Can you work these out from the model? Positions are in its coordinate system, mm. Face numbers are marked on the shaded views. A direction names the side the tool comes from. Give positions to 0.01 mm unless a question says otherwise; leave off trailing zeros. Order: outer loops, then holes, each group sorted by start corner. A loop starts at its lowest first (then second) coordinate and runs counter-clockwise, first axis right, second up. Notation, with made-up numbers: (87, -3.5) - (137, -3.5) arc R25 ccw to (137, 22.5) - close; hole circle Ø6 at (50.25, 7). An arc over 180 degrees is marked (long way). Answer as CSV lines item,"result".
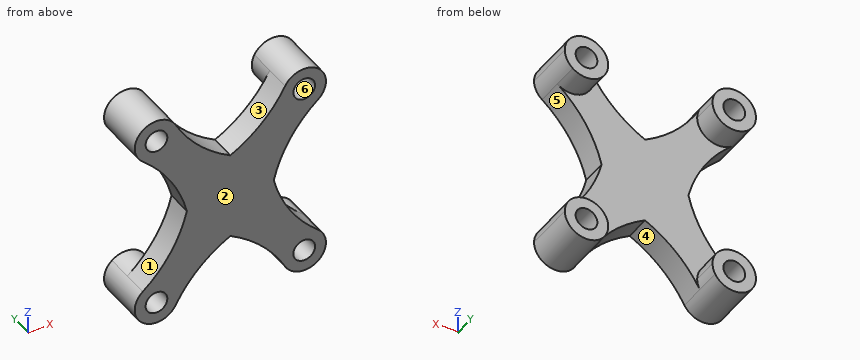
```python
from build123d import *

# Parameters (mm, degrees)
F0_R     = 2.5
F1_DEPTH = 12
F2_START = 6
F2_DEPTH = 6


# Not quite as in the source:
# - a feature names something its author has since deleted; it is built from what else it names


with BuildPart() as f1:
    # F0 (on Front) → F1 (new body)
    with BuildSketch(Plane.XZ):
        with BuildLine():
            ThreePointArc((-20.1639063661, 16.1283470576), (-14.8575168414, 15.4822831081), (-12, 20))
            ThreePointArc((-12, 20), (-12.1526927453, 21.2262187321), (-12.6014449516, 22.3775435823))
            ThreePointArc((-12.6014449516, 22.3775435823), (-20.1849966473, 23.8543217765), (-20.1639063661, 16.1283470576))
        make_face()
        with Locations((-17, 20)):
            Circle(F0_R, mode=Mode.SUBTRACT)
    extrude(amount=F1_DEPTH)



with BuildPart() as f1b:
    # F0 (on Front) → F1, piece 2 (new body)
    with BuildSketch(Plane.XZ):
        with BuildLine():
            ThreePointArc((22, 20), (18.2262187321, 24.8473072547), (12.6014449516, 22.3775435823))
            ThreePointArc((12.6014449516, 22.3775435823), (13.8150033527, 16.1456782235), (20.1639063661, 16.1283470576))
            ThreePointArc((20.1639063661, 16.1283470576), (21.5177168919, 17.8575168414), (22, 20))
        make_face()
        with Locations((17, 20)):
            Circle(F0_R, mode=Mode.SUBTRACT)
    extrude(amount=F1_DEPTH)


with BuildPart() as f1c:
    # F0 (on Front) → F1, piece 3 (new body)
    with BuildSketch(Plane.XZ):
        with BuildLine():
            ThreePointArc((22, -20), (21.5177168919, -17.8575168414), (20.1639063661, -16.1283470576))
            ThreePointArc((20.1639063661, -16.1283470576), (13.8150033527, -16.1456782235), (12.6014449516, -22.3775435823))
            ThreePointArc((12.6014449516, -22.3775435823), (18.2262187321, -24.8473072547), (22, -20))
        make_face()
        with Locations((17, -20)):
            Circle(F0_R, mode=Mode.SUBTRACT)
    extrude(amount=F1_DEPTH)


with BuildPart() as f1d:
    # F0 (on Front) → F1, piece 4 (new body)
    with BuildSketch(Plane.XZ):
        with BuildLine():
            ThreePointArc((-12, -20), (-14.8575168414, -15.4822831081), (-20.1639063661, -16.1283470576))
            ThreePointArc((-20.1639063661, -16.1283470576), (-20.1849966473, -23.8543217765), (-12.6014449516, -22.3775435823))
            ThreePointArc((-12.6014449516, -22.3775435823), (-12.1526927453, -21.2262187321), (-12, -20))
        make_face()
        with Locations((-17, -20)):
            Circle(F0_R, mode=Mode.SUBTRACT)
    extrude(amount=F1_DEPTH)


with BuildPart() as f1_1:
    add(f1.part)

    add(f1b.part)  # F2 merges F1b

    add(f1c.part)  # F2 merges F1c

    add(f1d.part)  # F2 merges F1d
    # F0 (on Front) → F2 (join)
    with BuildSketch(Plane.XZ.offset(F2_START)):
        with BuildLine():
            ThreePointArc((-12.6014449516, 22.3775435823), (-12.1526927453, 21.2262187321), (-12, 20))
            ThreePointArc((-12, 20), (-14.8575168414, 15.4822831081), (-20.1639063661, 16.1283470576))
            ThreePointArc((-20.1639063661, 16.1283470576), (-13.766762281, 8.8929923243), (-10, 0))
            ThreePointArc((-10, 0), (-7.0710678119, 7.0710678119), (0, 10))
            ThreePointArc((0, 10), (-7.2323271671, 15.2403150028), (-12.6014449516, 22.3775435823))
        make_face()
        with BuildLine():
            ThreePointArc((10, 0), (7.0710678119, 7.0710678119), (0, 10))
            ThreePointArc((0, 10), (-7.0710678119, 7.0710678119), (-10, 0))
            ThreePointArc((-10, 0), (-7.0710678119, -7.0710678119), (0, -10))
            ThreePointArc((0, -10), (7.0710678119, -7.0710678119), (10, 0))
        make_face()
        with BuildLine():
            ThreePointArc((0, -10), (-7.0710678119, -7.0710678119), (-10, 0))
            ThreePointArc((-10, 0), (-13.766762281, -8.8929923243), (-20.1639063661, -16.1283470576))
            ThreePointArc((-20.1639063661, -16.1283470576), (-14.8575168414, -15.4822831081), (-12, -20))
            ThreePointArc((-12, -20), (-12.1526927453, -21.2262187321), (-12.6014449516, -22.3775435823))
            ThreePointArc((-12.6014449516, -22.3775435823), (-7.2323271671, -15.2403150028), (0, -10))
        make_face()
        with BuildLine():
            ThreePointArc((20.1639063661, -16.1283470576), (13.766762281, -8.8929923243), (10, 0))
            ThreePointArc((10, 0), (7.0710678119, -7.0710678119), (0, -10))
            ThreePointArc((0, -10), (7.2323271671, -15.2403150028), (12.6014449516, -22.3775435823))
            ThreePointArc((12.6014449516, -22.3775435823), (13.8150033527, -16.1456782235), (20.1639063661, -16.1283470576))
        make_face()
        with BuildLine():
            ThreePointArc((12.6014449516, 22.3775435823), (7.2323271671, 15.2403150028), (0, 10))
            ThreePointArc((0, 10), (7.0710678119, 7.0710678119), (10, 0))
            ThreePointArc((10, 0), (13.766762281, 8.8929923243), (20.1639063661, 16.1283470576))
            ThreePointArc((20.1639063661, 16.1283470576), (13.8150033527, 16.1456782235), (12.6014449516, 22.3775435823))
        make_face()
    extrude(amount=F2_DEPTH)


solid = f1_1.part
```
1) I want a section at C-C on y = -8.5. Write out the boundary of the cut face in (x, z), plus the area to 3 significant figures.
Answer block:
outline,"(-20.16, -16.13) arc R5 ccw (long way) to (-12.6, -22.38) arc R30 cw to (0, -10) arc R30 cw to (12.6, -22.38) arc R5 ccw (long way) to (20.16, -16.13) arc R30 cw to (10, 0) arc R30 cw to (20.16, 16.13) arc R5 ccw (long way) to (12.6, 22.38) arc R30 cw to (0, 10) arc R30 cw to (-12.6, 22.38) arc R5 ccw (long way) to (-20.16, 16.13) arc R30 cw to (-10, 0) arc R30 cw to start; hole circle Ø5 at (-17, -20); hole circle Ø5 at (-17, 20); hole circle Ø5 at (17, -20); hole circle Ø5 at (17, 20)"
area,"1,050 mm2"
2) I want a section at D-D on z = 3. Write out the boundary of the cut face in (x, y).
Answer block:
outline,"(-10.9, -12) - (10.9, -12) - (10.9, -6) - (-10.9, -6) - close"
3) Which directions (+Z, -Z, +X, -X, +Y, -Y) give clear straight access to the entire face, cutting with the end or side of a thin tool? Please do the marked faces 4, 5 and 6.
Answer block:
face 4,"-Z, +Y, -Y"
face 5,"+X, +Y, -Y"
face 6,"+Y, -Y"
4) I'm going to push flat-ended pins straight in: P1, Ø6, axis at y = -5.5, z = -6, coming from the +X side; P2, Ø4, axis at x = -7.5, y = -10, coming from the -Z side; P3, Ø10, axis at x = -4, z = 12.5, coming from the +Y side; P4, Ø6, axis at x = -17, z = -20, coming from the -Y side. Where does each tip first touch, or does it pass through?
Answer block:
P1,"x = 13.81"
P2,"z = -17.73"
P3,"y = -6"
P4,"y = -12"
5) I want a section at B-B on x = -18.5. Write out the boundary of the cut face in (y, z), plus the area to 3 significant figures.
Answer block:
outline,"(-12, -24.77) - (0, -24.77) - (0, -22) - (-12, -22) - close; (-12, -18) - (0, -18) - (0, -15.23) - (-6, -15.23) - (-6, -14.66) - (-12, -14.66) - close; (-12, 14.66) - (-6, 14.66) - (-6, 15.23) - (0, 15.23) - (0, 18) - (-12, 18) - close; (-12, 22) - (0, 22) - (0, 24.77) - (-12, 24.77) - close"
area,"140 mm2"
6) If we mould it in two halves opening along Z, with no side actions, what happens to the marked faces 1, 2 and 3? For each: +Z half, -Z half, draft (parallel to the pull), parting line (faces both ways), or undercut.
Answer block:
face 1,"undercut"
face 2,"draft"
face 3,"+Z half"
7) I need wall thicknesses on line 1 along Z through (x, y) = (17, -5); line 2 along X through (y, z) = (-1.25, 22); line 3 along X through (y, z) = (-6.25, 19). Which ranges of each line are inside material? Lowest first, please. Write a range as [from, to].
Answer block:
line 1,"[-25, -22.5], [-17.5, -15], [15, 17.5], [22.5, 25]"
line 2,"[-21.58, -18.5], [-15.5, -12.42], [12.42, 15.5], [18.5, 21.58]"
line 3,"[-21.9, -19.29], [-14.71, -10.47], [10.47, 14.71], [19.29, 21.9]"
8) I want a section at A-A on y = -4.5. Write out the boundary of the cut face in (x, z), plus the area to 3 significant figures.
Answer block:
outline,"circle Ø10 at (-17, -20); circle Ø10 at (-17, 20); circle Ø10 at (17, -20); circle Ø10 at (17, 20); hole circle Ø5 at (-17, -20); hole circle Ø5 at (-17, 20); hole circle Ø5 at (17, -20); hole circle Ø5 at (17, 20)"
area,"236 mm2"
